from build123d import *

# Parameters (mm, degrees)
SKETCH1_R           = 1
SKETCH1_R_2         = 1.5
BOSS_EXTRUDE1_DEPTH = 2
CUT_EXTRUDE1_DEPTH  = 146.720996494
SKETCH3_W           = 5
SKETCH3_H           = 40
SKETCH3_W_2         = 20
SKETCH3_H_2         = 20
SKETCH3_W_3         = 28
SKETCH3_H_3         = 18
CUT_EXTRUDE2_DEPTH  = 2
SKETCH4_R           = 1
CUT_EXTRUDE3_DEPTH  = 2
SKETCH5_W           = 8
SKETCH5_H           = 1.5
SKETCH5_W_2         = 1.5
SKETCH5_H_2         = 8
BOSS_EXTRUDE2_DEPTH = 4


with BuildPart() as part:
    # Sketch1 → Boss-Extrude1 (new body)
    with BuildSketch(Plane.XY):
        Polygon((5.071460992, -3.5), (57.78242964, -3.5), (57.78242964, 130.260231922), (5.071460992, 130.260231922), (5.071460992, 125.260231922), (11.071460992, 125.260231922), (11.071460992, 2.5), (5.071460992, 2.5), align=None)
        with Locations((54.28242964, 0)):
            Circle(SKETCH1_R, mode=Mode.SUBTRACT)
        with Locations((54.28242964, 126.760231922)):
            Circle(SKETCH1_R, mode=Mode.SUBTRACT)
        with Locations((17.78242964, 70.260231922)):
            Circle(SKETCH1_R_2, mode=Mode.SUBTRACT)
    extrude(amount=BOSS_EXTRUDE1_DEPTH)

    # Sketch2 → Cut-Extrude1 (cut, through all)
    with BuildSketch(Plane.XZ.offset(3.5)):
        Polygon((6.036400554, 2.65114966), (1.157662204, -10.753073792), (3.527877144, 2.341321616), align=None)
    extrude(amount=-CUT_EXTRUDE1_DEPTH, mode=Mode.SUBTRACT)

    # Sketch3 → Cut-Extrude2 (cut)
    with BuildSketch(Plane.XY.offset(2)):
        with Locations((49.28242964, 46.5)):
            Rectangle(SKETCH3_W, SKETCH3_H)
        with Locations((21.071460992, 111.260231922)):
            Rectangle(SKETCH3_W_2, SKETCH3_H_2)
        with Locations((-0.078047732, 70.780115961)):
            Rectangle(SKETCH3_W_3, SKETCH3_H_3)
    extrude(amount=-CUT_EXTRUDE2_DEPTH, mode=Mode.SUBTRACT)

    # Sketch4 → Cut-Extrude3 (cut)
    with BuildSketch(Plane.XY.offset(2)):
        with Locations((17.38242964, 2.5)):
            Circle(SKETCH4_R)
        with Locations((42.78242964, 2.5)):
            Circle(SKETCH4_R)
        with Locations((42.78242964, 91.4)):
            Circle(SKETCH4_R)
        with Locations((17.38242964, 91.4)):
            Circle(SKETCH4_R)
    extrude(amount=-CUT_EXTRUDE3_DEPTH, mode=Mode.SUBTRACT)

    # Sketch5 → Boss-Extrude2 (add)
    with BuildSketch(Plane.XY.offset(2)):
        with Locations((18.78242964, 127.860231922)):
            Rectangle(SKETCH5_W, SKETCH5_H)
        with Locations((18.78242964, -1.1)):
            Rectangle(SKETCH5_W, SKETCH5_H)
        with Locations((55.38242964, 116.260231922)):
            Rectangle(SKETCH5_W_2, SKETCH5_H_2)
        with Locations((55.38242964, 10.5)):
            Rectangle(SKETCH5_W_2, SKETCH5_H_2)
    extrude(amount=-BOSS_EXTRUDE2_DEPTH)


solid = part.part
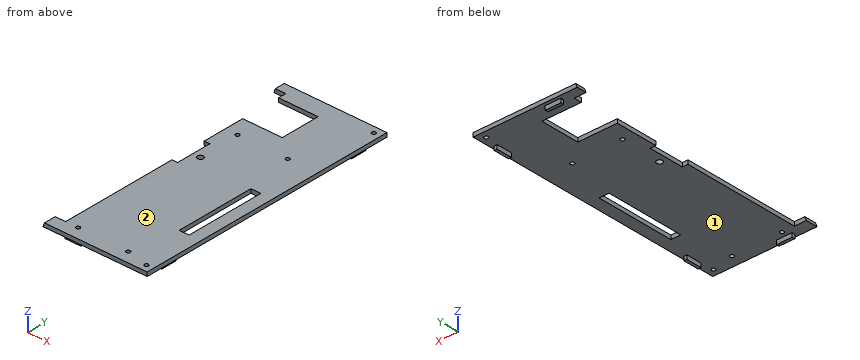
Input: part model. Units: mm. Frame: model coordinates. Face numbers are marked on the shaded views. Round coordinates to 2 decimals unless told otherwise and drop trailing zeros. Loops run counter-clockwise (first coordinate to the right, second up) from the corner with the lowest first, then second, coordinate; pieces in that order, holes last. Notation, with made-up numbers: M -38.75,84.5 L 5.25,84.5 A17 cw 5.25,97.5 Z; hole C 13,82.5 d7. An arc over 180 degrees is marked long. Answer as CSV lines item,"result". Start each with the question number.
(1) Section B-B, the plane y = 54. Output: boundary loops of the cut face in (x, z), plus the area to 3 significant figures.
(2) First-contact query: pin 1 (1.6 mm diameter, centred on y = 37.5, z = 1, fed in from -X); pin 2 (1 mm diameter, centred on x = 18, z = -1, fed in from +Y); pin 3 (2 mm diameter, centred on y = 117.5, z = -1.5, fed in from -X). Flat tips, straight axial feed; report the tip coordinate or a pass-through.
(3) Section D-D, the plane x = 39. Output: boundary loops of the cut face in (y, z), plus the area to 3 significant figures.
(4) Section A-A, the plane z = -0.8. Output: boundary loops of the cut face in (x, y).
(5) Section C-C, the plane x = 49. Output: boundary loops of the cut face in (y, z), plus the area to 3 significant figures.
(6) Line query: line 1 (X direction, y = 91.4, z = 0.6); line 2 (Y direction, x = 22.5, z = -1.45); line 3 (Y direction, x = 30.5, z = 1.3). Output: solid intervals per line, ascending. Write a range as [from, to].
(7) Draft query along Y for the marked faces 1 and 2. Return one class per face: released by +Y, released by -Y, zero draft, split by the parting line, or undercut.
Values found:
1,outline,"M 11.07,0 L 46.78,0 L 46.78,2 L 11.07,2 Z; M 51.78,0 L 57.78,0 L 57.78,2 L 51.78,2 Z"
1,area,"83.4 mm²"
2,pin 1,"stops at x = 11.07"
2,pin 2,"stops at y = 128.61"
2,pin 3,"stops at x = 54.63"
3,outline,"M -3.5,0 L 130.26,0 L 130.26,2 L -3.5,2 Z"
3,area,"268 mm²"
4,outline,"M 14.78,-1.85 L 22.78,-1.85 L 22.78,-0.35 L 14.78,-0.35 Z; M 14.78,127.11 L 22.78,127.11 L 22.78,128.61 L 14.78,128.61 Z; M 54.63,6.5 L 56.13,6.5 L 56.13,14.5 L 54.63,14.5 Z; M 54.63,112.26 L 56.13,112.26 L 56.13,120.26 L 54.63,120.26 Z"
5,outline,"M -3.5,0 L 26.5,0 L 26.5,2 L -3.5,2 Z; M 66.5,0 L 130.26,0 L 130.26,2 L 66.5,2 Z"
5,area,"188 mm²"
6,line 1,"x = [11.07, 16.38], [18.38, 41.78], [43.78, 57.78]"
6,line 2,"y = [-1.85, -0.35], [127.11, 128.61]"
6,line 3,"y = [-3.5, 101.26], [121.26, 130.26]"
7,face 1,"undercut"
7,face 2,"zero draft"
